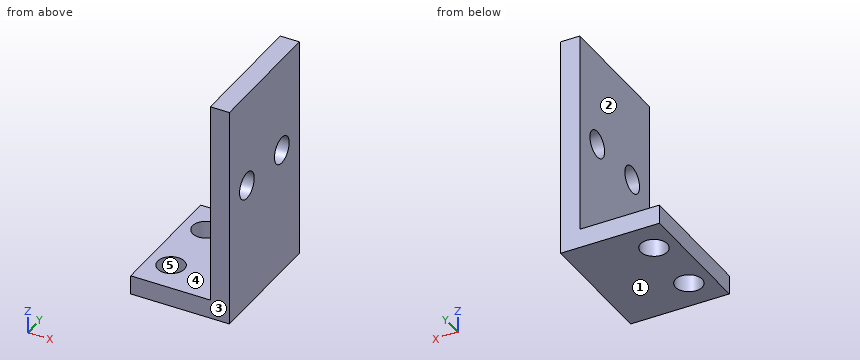
from build123d import *

# Parameters (mm, degrees)
SKETCH_1_W                  = 20
SKETCH_1_H                  = 35
EXTRUDE_1_DEPTH             = 15.5
SKETCH_2_W                  = 12.5
SKETCH_2_H                  = 32
CUT_EXTRUDE_1_DEPTH         = 49.176757882
HOLE_WIZARD_4_2_4_2_1_D     = 4.2
HOLE_WIZARD_4_2_4_2_1_DEPTH = 15.5
HOLE_WIZARD_4_2_4_2_2_D     = 4.2


with BuildPart() as part:
    # 草图1 → 凸台-拉伸1 (new body)
    with BuildSketch(Plane(origin=(20.5, 0, 0), x_dir=(0, -1, 0), z_dir=(-1, 0, 0))):
        with Locations((40, 7.5)):
            Rectangle(SKETCH_1_W, SKETCH_1_H)
    extrude(amount=-EXTRUDE_1_DEPTH)

    # 草图2 → 切除-拉伸1 (cut, through all)
    with BuildSketch(Plane.XZ.offset(50)):
        with Locations((26.75, 9)):
            Rectangle(SKETCH_2_W, SKETCH_2_H)
    extrude(amount=-CUT_EXTRUDE_1_DEPTH, mode=Mode.SUBTRACT)

    # Ø4.2 (4.2) 直径孔1
    with Locations(Plane(origin=(36, 0, 0), x_dir=(0, 0, -1), z_dir=(1, 0, 0))):
        with Locations((-10, -35), (-10, -45)):
            Hole(HOLE_WIZARD_4_2_4_2_1_D / 2, depth=HOLE_WIZARD_4_2_4_2_1_DEPTH)

    # Ø4.2 (4.2) 直径孔2 (through all)
    with Locations(Plane.XY.offset(-7)):
        with Locations((24.1, -45), (24.1, -35)):
            Hole(HOLE_WIZARD_4_2_4_2_2_D / 2)


solid = part.part
Build history of the part. All positions in model axes, mm. Face numbers are marked on the shaded views. A direction names the side the tool comes from. Round coordinates to 2 decimals unless told otherwise and drop trailing zeros. Loops run counter-clockwise (first coordinate to the right, second up) from the corner with the lowest first, then second, coordinate; pieces in that order, holes last. Notation, with made-up numbers: (46.25, 57) -> (87.25, 57) arc R16 ccw to (87.25, 76) -> close; hole circle Ø8 at (84.5, 59.5). An arc over 180 degrees is marked (long way). Use CSV: the item, a comma, the result in double quotes. Start each with the question number.
Q1. Saw through at A-A on z = 10. Give the cut face in (x, y), and give its area (3 significant figures).
Q2. Which spindle directions (+Z, -Z, +X, -X, +Y, -Y) get a long thin tool onto all of the face, cutting with end or side? Do the marked faces 1 and 2. Say none if no direction does.
Q3. Flat gauge pins, fed straight in: pin 1 Ø6 at (x, y) = (28, -38.5) entering from +Z; pin 2 Ø5 at (y, z) = (-45, 10) entering from -X; pin 3 Ø5 at (x, y) = (31.5, -44) entering from +Z. Where does each tip first touch, or does it go through?
Q4. Saw through at D-D on x = 33.5. Give the cut face in (y, z), and give its area (3 significant figures).
Q5. Drill centre lines: L1, parallel to Y at x = 34, z = 10; L2, parallel to Z at x = 21.5, y = -37; L3, parallel to X at y = -34.5, z = 1. Where is each one in solid material? Low to high.
Q6. Saw through at C-C on x = 24.1. Give the cut face in (y, z).
Q7. Mould opens along Y. For the marked faces 3, 4 and 5 say: +Y half, -Y half, draft (parallel to the pull), parting line (faces both ways), or undercut.
Q8. Saw through at B-B on y = -45. Give the cut face in (x, z).
Solutions:
1,outline,"(33, -50) -> (36, -50) -> (36, -47.1) -> (33, -47.1) -> close; (33, -42.9) -> (36, -42.9) -> (36, -37.1) -> (33, -37.1) -> close; (33, -32.9) -> (36, -32.9) -> (36, -30) -> (33, -30) -> close"
1,area,"34.8 mm^2"
2,face 1,"-Z, +X, -X, +Y, -Y"
2,face 2,"+Z, -X, +Y, -Y"
3,pin 1,"stops at z = -7"
3,pin 2,"stops at x = 33"
3,pin 3,"stops at z = 25"
4,outline,"(-50, -10) -> (-30, -10) -> (-30, 25) -> (-50, 25) -> close; hole circle Ø4.2 at (-45, 10); hole circle Ø4.2 at (-35, 10)"
4,area,"672 mm^2"
5,L1,"y = -50 to -47.1, -42.9 to -37.1, -32.9 to -30"
5,L2,"z = -10 to -7"
5,L3,"x = 33 to 36"
6,outline,"(-50, -10) -> (-47.1, -10) -> (-47.1, -7) -> (-50, -7) -> close; (-42.9, -10) -> (-37.1, -10) -> (-37.1, -7) -> (-42.9, -7) -> close; (-32.9, -10) -> (-30, -10) -> (-30, -7) -> (-32.9, -7) -> close"
7,face 3,"-Y half"
7,face 4,"draft"
7,face 5,"undercut"
8,outline,"(20.5, -10) -> (22, -10) -> (22, -7) -> (20.5, -7) -> close; (26.2, -10) -> (36, -10) -> (36, 7.9) -> (33, 7.9) -> (33, -7) -> (26.2, -7) -> close; (33, 12.1) -> (36, 12.1) -> (36, 25) -> (33, 25) -> close"
